```python
from build123d import *

# Parameters (mm, degrees)
BOSS_EXTRUDE1_DEPTH      = 9
BOSS_EXTRUDE1_DEPTH_BACK = 28
SKETCH1_R                = 18
SKETCH2_W                = 50.00806526
SKETCH2_H                = 20.388963247
CUT_EXTRUDE1_DEPTH       = 137
SKETCH6_R                = 2.56681782
CUT_EXTRUDE2_DEPTH       = 40
BOSS_EXTRUDE2_START      = 170
SKETCH7_W                = 42.331288986
SKETCH7_H                = 30
BOSS_EXTRUDE2_DEPTH      = 4
FILLET1_R                = 10


with BuildPart() as part:
    # Sketch1 → Boss-Extrude1 (new, two sides: drawn at the far end of the back side and taken through both)
    with BuildSketch(Plane(origin=(0, 0, 126.356389087), x_dir=(-1, 0, 0), z_dir=(0, 0, -1)).offset(-BOSS_EXTRUDE1_DEPTH_BACK)):
        with Locations((-188.724341924, 64.165727937)):
            Circle(SKETCH1_R)
    extrude(amount=BOSS_EXTRUDE1_DEPTH + BOSS_EXTRUDE1_DEPTH_BACK)

    # Sketch2 → Cut-Extrude1 (cut)
    with BuildSketch(Plane(origin=(-6.948170377, -29.446447031, 0), x_dir=(0.99748757373397, -0.07084165615171512, 3.115559675779194e-15), z_dir=(0.07084165615171512, 0.99748757373397, 0))):
        with Locations((192.53019978, -136.066593827)):
            Rectangle(SKETCH2_W, SKETCH2_H)
    extrude(amount=CUT_EXTRUDE1_DEPTH, mode=Mode.SUBTRACT)


with BuildPart() as cut_extrude1_piece_1:
    # of the separate pieces the step leaves, piece 1, a body of its own (cut_extrude1_pieces)
    add(part.part.solids().sort_by_distance((170.724341924, 64.165727937, 125.872112203))[0])


with BuildPart() as cut_extrude1_piece_2:
    # of the separate pieces the step leaves, piece 2, a body of its own (cut_extrude1_pieces)
    add(part.part.solids().sort_by_distance((170.724341924, 64.165727937, 146.26107545))[0])


with BuildPart() as cut_extrude2_tool:
    # Sketch6 → Cut-Extrude2 (new body)
    with BuildSketch(Plane(origin=(0, 0, 117.356389087), x_dir=(-1, 0, 0), z_dir=(0, 0, -1))):
        with Locations((-188.724341924, 64.165727937)):
            Circle(SKETCH6_R)
    extrude(amount=-CUT_EXTRUDE2_DEPTH)


with BuildPart() as cut_extrude1_piece_1_1:
    add(cut_extrude1_piece_1.part)

    # Cut-Extrude2: cut by cut_extrude2_tool
    add(cut_extrude2_tool.part, mode=Mode.SUBTRACT)



with BuildPart() as cut_extrude1_piece_2_1:
    add(cut_extrude1_piece_2.part)

    # Cut-Extrude2: cut by cut_extrude2_tool
    add(cut_extrude2_tool.part, mode=Mode.SUBTRACT)


with BuildPart() as cut_extrude1_piece_1_2:
    add(cut_extrude1_piece_1_1.part)

    add(cut_extrude1_piece_2_1.part)  # Boss-Extrude2 merges Cut-Extrude1 piece 2
    # Sketch7 → Boss-Extrude2 (add)
    with BuildSketch(Plane(origin=(0, 0, 0), x_dir=(0, 0, -1), z_dir=(1, 0, 0)).offset(BOSS_EXTRUDE2_START)):
        with Locations((-135.980164786, 63.44621419)):
            Rectangle(SKETCH7_W, SKETCH7_H)
    extrude(amount=BOSS_EXTRUDE2_DEPTH)

    # Fillet1
    # the kernel refuses this fillet: 10 mm, written as the material it adds along each edge
    with BuildSketch(Plane(origin=(174, 37.158405517, 117.356389087), x_dir=(0, 0, -1), z_dir=(0, 1, 0))) as fillet1_piece_1_section:
        with BuildLine():
            CenterArc((10, -6.66155229), FILLET1_R, 138.228987443, 41.771012557)
            Line((0, -6.66155229), (-0.2, -6.66155229))
            Line((-0.2, -6.66155229), (-0.2, 0))
            Line((-0.2, 0), (0, 0.2))
            ThreePointArc((0, 0.2), (1.270934397, 0.2), (2.39270617, 0.133231046))
            Line((2.39270617, 0.133231046), (2.541868794, 0))
        make_face()
    fillet1_piece_1 = extrude(amount=54.01464484, mode=Mode.PRIVATE)
    fillet1_piece_1 = fillet1_piece_1 & Plane(origin=(188.724341924, 64.165727937, 117.454219773), x_dir=(-1, 0, 0), z_dir=(0, 0, 1)) * Cylinder(18, 135, mode=Mode.PRIVATE)
    add(fillet1_piece_1)
    with BuildSketch(Plane(origin=(174, 36.49041805, 154.356389087), x_dir=(0, 0, 1), z_dir=(0, 1, 0))) as fillet1_piece_2_section:
        with BuildLine():
            CenterArc((10, 6.928747277), FILLET1_R, 180, 43.858101489)
            Line((0, 6.928747277), (-0.2, 6.928747277))
            Line((-0.2, 6.928747277), (-0.2, 0))
            Line((-0.2, 0), (0, -0.2))
            ThreePointArc((0, -0.2), (1.394710096, -0.2), (2.645208596, -0.138574946))
            Line((2.645208596, -0.138574946), (2.789420192, 0))
        make_face()
    fillet1_piece_2 = extrude(amount=55.350619773, mode=Mode.PRIVATE)
    fillet1_piece_2 = fillet1_piece_2 & Plane(origin=(188.724341924, 64.165727937, 154.260633817), x_dir=(-1, 0, 0), z_dir=(0, 0, -1)) * Cylinder(18, 139, mode=Mode.PRIVATE)
    add(fillet1_piece_2)


solid = cut_extrude1_piece_1_2.part
```
Verification items for the finished model (mm, model axes). A direction names the side the tool comes from. Give positions to 0.01 mm unless a question says otherwise; leave off trailing zeros. Write each loop counter-clockwise with the first axis right and the second up, starting at its lowest first coordinate (ties: lowest second). Pieces come first, ordered by that corner, then holes. Notation, with made-up numbers: M 67.25,9.5 L 115.25,9.5 A22 cw 115.25,30.5 Z; hole C 81,69 d10. An arc over 180 degrees is marked long. One line per question, with ' | ' between items.
1) Section check D-D on z = 137. Enter the section's corners in (x, y), plus the area to 3 significant figures.
Result:
outline: M 170,48.45 L 174,48.45 L 174,78.45 L 170,78.45 Z | area: 120 mm2
2) Thickness scan on line 1 along Z through (x, y) = (182.5, 78); line 2 along X through (y, z) = (51, 139); line 3 along X through (y, z) = (73, 121). Record the ranges inside material, lowest first. Write a range as [from, to].
Result:
line 1: z = [117.36, 125.87], [146.26, 154.36] | line 2: x = [170, 174] | line 3: x = [170, 204.41]
3) Set-up check for faces 5 (the flat face through (186, 64, 125.872)), 6 (the flat face through (172, 48.446, 136)), 7 (the flat face through (194, 64, 154.356)), 8 (the flat face through (194, 64, 117.356)): record each of +Z, -Z, +X, -X, +Y, -Y from which the full face is reachable in a straight line by a thin tool's end or side.
Result:
face 5: +X, +Y, -Y | face 6: +Z, -Z, -X, -Y | face 7: +Z, +X, +Y, -Y | face 8: -Z, +X, +Y, -Y
4) Section check A-A on x = 183.5. Enter the section's corners in (y, z), plus the area to 3 significant figures.
Result:
outline: M 46.94,117.36 L 81.39,117.36 L 81.39,125.87 L 46.94,125.87 Z; M 46.94,146.26 L 81.39,146.26 L 81.39,154.36 L 46.94,154.36 Z | area: 572 mm2
5) Gauge pin test, flat ends, axial feed: pin 1 Ø10 at (x, y) = (175.5, 76.5) entering from -Z; pin 2 Ø3 at (x, z) = (180.5, 145.5) entering from -Y; pin 3 Ø1 at (x, y) = (197.5, 57) entering from -Z; pin 4 Ø20.5 at (x, y) = (200, 73) entering from +Z. Record the tip position at first contact, or that the pin passes through.
Result:
pin 1: stops at z = 114.81 | pin 2: stops at y = 47.55 | pin 3: stops at z = 117.36 | pin 4: stops at z = 154.36
6) Section check B-B on y = 53. Enter the section's corners in (x, z).
Result:
outline: M 170,114.81 L 174,114.81 L 174,157.15 L 170,157.15 Z; M 174.61,115.31 A10 cw 180.66,117.36 L 202.84,117.36 L 202.84,125.87 L 174.61,125.87 Z; M 174.61,146.26 L 202.84,146.26 L 202.84,154.36 L 180.93,154.36 A10 cw 174.61,156.61 Z
7) Mould release check, pull along Z, two halves, no side actions. Record for faces 1 (the flat face through (186, 64, 146.261)), 2 (the flat face through (174, 64, 136)), 3 (the flat face through (172, 78.446, 136)), 4 (the flat face through (172, 63, 157.146)): released by +Z, released by -Z, zero draft, split by the parting line, or undercut.
Result:
face 1: undercut | face 2: undercut | face 3: zero draft | face 4: released by +Z
8) Section check C-C on z = 149.5. Enter the section's corners in (x, y), plus the area to 3 significant figures.
Result:
outline: M 170,48.45 L 174,48.45 L 174,53.81 A18 ccw long 174,74.52 L 174,78.45 L 170,78.45 Z; hole C 188.72,64.17 d5.13 | area: 1,070 mm2
